```python
from build123d import *

# Parameters (mm, degrees)
SKETCH2_R           = 14
BOSS_EXTRUDE2_DEPTH = 2.2
SKETCH3_R           = 12.5
BOSS_EXTRUDE5_DEPTH = 3.2
SKETCH4_R           = 6.75
BOSS_EXTRUDE6_DEPTH = 5.2
FILLET1_R           = 0.4


with BuildPart() as part:
    # Sketch2 → Boss-Extrude2 (new body)
    with BuildSketch(Plane.XY):
        Circle(SKETCH2_R)
    extrude(amount=BOSS_EXTRUDE2_DEPTH)

    # Sketch3 → Boss-Extrude5 (add)
    with BuildSketch(Plane.XY):
        Circle(SKETCH3_R)
    extrude(amount=BOSS_EXTRUDE5_DEPTH)

    # Sketch4 → Boss-Extrude6 (add)
    with BuildSketch(Plane.XY):
        Circle(SKETCH4_R)
    extrude(amount=BOSS_EXTRUDE6_DEPTH)

    # Fillet1
    fillet1_edges = [part.edges().sort_by_distance(p)[0] for p in [
        (-6.75, 0, 5.2),
        (-14, 0, 2.2),
        (-12.5, 0, 3.2),
    ]]
    fillet(fillet1_edges, radius=FILLET1_R)


solid = part.part
```
Verification items for the finished model (mm, model axes). A direction names the side the tool comes from. Give positions to 0.01 mm unless a question says otherwise; leave off trailing zeros. Order: outer loops, then holes, each group sorted by start corner. A loop starts at its lowest first (then second) coordinate and runs counter-clockwise, first axis right, second up. Notation, with made-up numbers: M 48,38 L 56,38 A8 ccw 56,52 Z; hole C 84.25,-15 d10. An arc over 180 degrees is marked long. Answer in a Markdown table with one row per item. Add a question column.
Item 1: Scan lines: probe 1 along Z at (x, y) = (-3, -11.5); probe 2 along X at (y, z) = (-5, 2.95); probe 3 along X at (y, z) = (-4, 1.4). Record each from-to range of solid material in increasing order. Write a range as from..to.
Item 2: Section check D-D, the plane z = 0.4. Enter the section's corners in (x, y).
Item 3: Section check C-C, the plane z = 3.7. Enter the section's corners in (x, y), and give its area (3 significant figures).
Item 4: Gauge pin test, flat ends, axial feed: pin 1 (3 mm diameter, centred on y = -3.5, z = 1.5, fed in from +X); pin 2 (2 mm diameter, centred on x = -5, z = 1, fed in from +Y); pin 3 (5 mm diameter, centred on x = -7.5, y = 8, fed in from +Z). Record the tip position at first contact, or that the pin passes through.
Item 5: Tool access check on faces 1 (the flat face through (0, 0, 0)), 2 (the cylindrical face through (-1.46, -6.59, 3.99)). Record the directions out of +Z, -Z, +X, -X, +Y, -Y that give a thin tool (end or side, any length) a straight path to the whole face; none if there is none.
Item 6: Section check A-A, the plane y = 0. Enter the section's corners in (x, z).
Filled sheet:
| question | item | result |
|---|---|---|
| 1 | probe 1 | z = 0..3.2 |
| 1 | probe 2 | x = -11.42..11.42 |
| 1 | probe 3 | x = -13.42..13.42 |
| 2 | outline | C 0,0 d28 |
| 3 | outline | C 0,0 d13.5 |
| 3 | area | 143 mm^2 |
| 4 | pin 1 | stops at x = 13.86 |
| 4 | pin 2 | stops at y = 13.42 |
| 4 | pin 3 | stops at z = 3.2 |
| 5 | face 1 | -Z, +X, -X, +Y, -Y |
| 5 | face 2 | +Z |
| 6 | outline | M -14,0 L 14,0 L 14,1.8 A0.4 ccw 13.6,2.2 L 12.5,2.2 L 12.5,2.8 A0.4 ccw 12.1,3.2 L 6.75,3.2 L 6.75,4.8 A0.4 ccw 6.35,5.2 L -6.35,5.2 A0.4 ccw -6.75,4.8 L -6.75,3.2 L -12.1,3.2 A0.4 ccw -12.5,2.8 L -12.5,2.2 L -13.6,2.2 A0.4 ccw -14,1.8 Z |
